For this review, take the finished solid that the model builds, in its own axes (mm). A direction names the side the tool comes from. Give positions to 0.01 mm unless a question says otherwise; leave off trailing zeros. Write each loop counter-clockwise with the first axis right and the second up, starting at its lowest first coordinate (ties: lowest second). Pieces come first, ordered by that corner, then holes. Notation, with made-up numbers: (85, 69) -> (143, 69) arc R26 cw to (143, 108) -> close; hole circle Ø7 at (18, -33). An arc over 180 degrees is marked (long way). Return JSON: item names as keys, results as strings.
from build123d import *

# Parameters (mm, degrees)
F2_R            = 12.5
F3_DEPTH        = 6
F5_DEPTH        = 68
F6_R            = 12.5
F7_DEPTH        = 12
F8_DEPTH        = 6
F12_D           = 8
F12_DEPTH       = 25
F12_CSINK_D     = 12
F12_CSINK_ANGLE = 60
F12_TIP         = 2.4034424761
F14_DEPTH       = 33
F15_R           = 9
F15_R_2         = 8.5
F16_DEPTH       = 6


with BuildPart() as f1:
    # F0 (on Front) → F1 (revolve)
    with BuildSketch(Plane.XZ):
        Polygon((0, 10), (0, 0), (86.0796358759, 0), (86.0796358759, 8), (85.0796358759, 9), (52.7846625228, 9), (52.7846625228, 8.5), (46, 8.5), (46, 10), align=None)
    revolve(axis=Axis((43.0398179379, 0, 0), (-1, 0, 0)))

    # F2 (on face) → F3 (join)
    with BuildSketch(Plane(origin=(0, 0, 0), x_dir=(0, -1, 0), z_dir=(-1, 0, 0))):
        Circle(F2_R)
    extrude(amount=F3_DEPTH)

    # F4 (on face) → F5 (join)
    with BuildSketch(Plane(origin=(-6, 0, 0), x_dir=(0, -1, 0), z_dir=(-1, 0, 0))):
        with BuildLine():
            Line((8.0269876576, 7.5211348309), (6.2374895659, 6.4879676259))
            ThreePointArc((6.2374895659, 6.4879676259), (4.5, 7.7942286341), (2.5, 8.6458082329))
            Line((2.5, 8.6458082329), (2.5, 10.7121426428))
            ThreePointArc((2.5, 10.7121426428), (0, 11), (-2.5, 10.7121426428))
            Line((-2.5, 10.7121426428), (-2.5, 8.6458082329))
            ThreePointArc((-2.5, 8.6458082329), (-4.5, 7.7942286341), (-6.2374895659, 6.4879676259))
            Line((-6.2374895659, 6.4879676259), (-8.0269876576, 7.5211348309))
            ThreePointArc((-8.0269876576, 7.5211348309), (-9.5262794416, 5.5), (-10.5269876576, 3.1910078119))
            Line((-10.5269876576, 3.1910078119), (-8.7374895659, 2.157840607))
            ThreePointArc((-8.7374895659, 2.157840607), (-9, 0), (-8.7374895659, -2.157840607))
            Line((-8.7374895659, -2.157840607), (-10.5269876576, -3.1910078119))
            ThreePointArc((-10.5269876576, -3.1910078119), (-9.5262794416, -5.5), (-8.0269876576, -7.5211348309))
            Line((-8.0269876576, -7.5211348309), (-6.2374895659, -6.4879676259))
            ThreePointArc((-6.2374895659, -6.4879676259), (-4.5, -7.7942286341), (-2.5, -8.6458082329))
            Line((-2.5, -8.6458082329), (-2.5, -10.7121426428))
            ThreePointArc((-2.5, -10.7121426428), (0, -11), (2.5, -10.7121426428))
            Line((2.5, -10.7121426428), (2.5, -8.6458082329))
            ThreePointArc((2.5, -8.6458082329), (4.5, -7.7942286341), (6.2374895659, -6.4879676259))
            Line((6.2374895659, -6.4879676259), (8.0269876576, -7.5211348309))
            ThreePointArc((8.0269876576, -7.5211348309), (9.5262794416, -5.5), (10.5269876576, -3.1910078119))
            Line((10.5269876576, -3.1910078119), (8.7374895659, -2.157840607))
            ThreePointArc((8.7374895659, -2.157840607), (9, 0), (8.7374895659, 2.157840607))
            Line((8.7374895659, 2.157840607), (10.5269876576, 3.1910078119))
            ThreePointArc((10.5269876576, 3.1910078119), (10.0928807369, 4.3742151788), (9.5262794416, 5.5))
            ThreePointArc((9.5262794416, 5.5), (8.8346218349, 6.5535835262), (8.0269876576, 7.5211348309))
        make_face()
    extrude(amount=F5_DEPTH)

    # F6 (on face) → F7 (cut)
    with BuildSketch(Plane(origin=(-6, 0, 0), x_dir=(0, -1, 0), z_dir=(-1, 0, 0))):
        Circle(F6_R)
        with BuildLine():
            ThreePointArc((2.5, 8.6458082329), (4.5, 7.7942286341), (6.2374895659, 6.4879676259))
            Line((6.2374895659, 6.4879676259), (8.0269876576, 7.5211348309))
            ThreePointArc((8.0269876576, 7.5211348309), (9.5262794416, 5.5), (10.5269876576, 3.1910078119))
            Line((10.5269876576, 3.1910078119), (8.7374895659, 2.157840607))
            ThreePointArc((8.7374895659, 2.157840607), (9, 0), (8.7374895659, -2.157840607))
            Line((8.7374895659, -2.157840607), (10.5269876576, -3.1910078119))
            ThreePointArc((10.5269876576, -3.1910078119), (9.5262794416, -5.5), (8.0269876576, -7.5211348309))
            Line((8.0269876576, -7.5211348309), (6.2374895659, -6.4879676259))
            ThreePointArc((6.2374895659, -6.4879676259), (4.5, -7.7942286341), (2.5, -8.6458082329))
            Line((2.5, -8.6458082329), (2.5, -10.7121426428))
            ThreePointArc((2.5, -10.7121426428), (0, -11), (-2.5, -10.7121426428))
            Line((-2.5, -10.7121426428), (-2.5, -8.6458082329))
            ThreePointArc((-2.5, -8.6458082329), (-4.5, -7.7942286341), (-6.2374895659, -6.4879676259))
            Line((-6.2374895659, -6.4879676259), (-8.0269876576, -7.5211348309))
            ThreePointArc((-8.0269876576, -7.5211348309), (-9.5262794416, -5.5), (-10.5269876576, -3.1910078119))
            Line((-10.5269876576, -3.1910078119), (-8.7374895659, -2.157840607))
            ThreePointArc((-8.7374895659, -2.157840607), (-9, 0), (-8.7374895659, 2.157840607))
            Line((-8.7374895659, 2.157840607), (-10.5269876576, 3.1910078119))
            ThreePointArc((-10.5269876576, 3.1910078119), (-9.5262794416, 5.5), (-8.0269876576, 7.5211348309))
            Line((-8.0269876576, 7.5211348309), (-6.2374895659, 6.4879676259))
            ThreePointArc((-6.2374895659, 6.4879676259), (-4.5, 7.7942286341), (-2.5, 8.6458082329))
            Line((-2.5, 8.6458082329), (-2.5, 10.7121426428))
            ThreePointArc((-2.5, 10.7121426428), (0, 11), (2.5, 10.7121426428))
            Line((2.5, 10.7121426428), (2.5, 8.6458082329))
        make_face(mode=Mode.SUBTRACT)
    extrude(amount=-F7_DEPTH, mode=Mode.SUBTRACT)

    # F6 (on face) → F8 (join)
    with BuildSketch(Plane(origin=(-6, 0, 0), x_dir=(0, -1, 0), z_dir=(-1, 0, 0))):
        Circle(F6_R)
        with BuildLine():
            ThreePointArc((2.5, 8.6458082329), (4.5, 7.7942286341), (6.2374895659, 6.4879676259))
            Line((6.2374895659, 6.4879676259), (8.0269876576, 7.5211348309))
            ThreePointArc((8.0269876576, 7.5211348309), (9.5262794416, 5.5), (10.5269876576, 3.1910078119))
            Line((10.5269876576, 3.1910078119), (8.7374895659, 2.157840607))
            ThreePointArc((8.7374895659, 2.157840607), (9, 0), (8.7374895659, -2.157840607))
            Line((8.7374895659, -2.157840607), (10.5269876576, -3.1910078119))
            ThreePointArc((10.5269876576, -3.1910078119), (9.5262794416, -5.5), (8.0269876576, -7.5211348309))
            Line((8.0269876576, -7.5211348309), (6.2374895659, -6.4879676259))
            ThreePointArc((6.2374895659, -6.4879676259), (4.5, -7.7942286341), (2.5, -8.6458082329))
            Line((2.5, -8.6458082329), (2.5, -10.7121426428))
            ThreePointArc((2.5, -10.7121426428), (0, -11), (-2.5, -10.7121426428))
            Line((-2.5, -10.7121426428), (-2.5, -8.6458082329))
            ThreePointArc((-2.5, -8.6458082329), (-4.5, -7.7942286341), (-6.2374895659, -6.4879676259))
            Line((-6.2374895659, -6.4879676259), (-8.0269876576, -7.5211348309))
            ThreePointArc((-8.0269876576, -7.5211348309), (-9.5262794416, -5.5), (-10.5269876576, -3.1910078119))
            Line((-10.5269876576, -3.1910078119), (-8.7374895659, -2.157840607))
            ThreePointArc((-8.7374895659, -2.157840607), (-9, 0), (-8.7374895659, 2.157840607))
            Line((-8.7374895659, 2.157840607), (-10.5269876576, 3.1910078119))
            ThreePointArc((-10.5269876576, 3.1910078119), (-9.5262794416, 5.5), (-8.0269876576, 7.5211348309))
            Line((-8.0269876576, 7.5211348309), (-6.2374895659, 6.4879676259))
            ThreePointArc((-6.2374895659, 6.4879676259), (-4.5, 7.7942286341), (-2.5, 8.6458082329))
            Line((-2.5, 8.6458082329), (-2.5, 10.7121426428))
            ThreePointArc((-2.5, 10.7121426428), (0, 11), (2.5, 10.7121426428))
            Line((2.5, 10.7121426428), (2.5, 8.6458082329))
        make_face(mode=Mode.SUBTRACT)
    extrude(amount=-F8_DEPTH)

    # F9 (on Front) → F10 (revolve)
    with BuildSketch(Plane.XZ):
        Polygon((-92, 0), (-74, 0), (-74, 2.157840607), (-74, 3.1910078119), (-74, 7.5211348309), (-74, 8.3), (-76, 8.3), (-76, 8.5), (-91, 8.5), (-92, 7.5), align=None)
    revolve(axis=Axis((-83, 0, 0), (1, 0, 0)))

    # F12
    with Locations(Plane.YZ.offset(86.0796358759)):
        with Locations((0, 0)):
            CounterSinkHole(F12_D / 2, F12_CSINK_D / 2, depth=F12_DEPTH, counter_sink_angle=F12_CSINK_ANGLE)
            with Locations((0, 0, -(F12_DEPTH + F12_TIP / 2))):  # 118° drill point
                Cone(0, F12_D / 2, F12_TIP, mode=Mode.SUBTRACT)

    # F13 (on face) → F14 (cut)
    with BuildSketch(Plane.YZ.offset(86.0796358759)):
        with BuildLine():
            Line((-2.5, 7), (0, 7))
            Line((0, 7), (2.5, 7))
            Line((2.5, 7), (2.5, 8.6458082329))
            ThreePointArc((2.5, 8.6458082329), (0, 9), (-2.5, 8.6458082329))
            Line((-2.5, 8.6458082329), (-2.5, 7))
        make_face()
    extrude(amount=-F14_DEPTH, mode=Mode.SUBTRACT)

    # F15 (on face) → F16 (join)
    with BuildSketch(Plane(origin=(52.7846625228, 0, 0), x_dir=(0, -1, 0), z_dir=(-1, 0, 0))):
        Circle(F15_R)
        Circle(F15_R_2, mode=Mode.SUBTRACT)
    extrude(amount=F16_DEPTH)


solid = f1.part
1. Add section A-A, the plane x = 73. State the section outline as (y, z) points, plus the area to 3 significant figures.
Results found:
{"outline": "(-2.5, 7) -> (-2.5, 8.65) arc R9 ccw (long way) to (2.5, 8.65) -> (2.5, 7) -> close; hole circle Ø8 at (0, 0)", "area": "195 mm²"}
2. To check wall thickness, follow probe 1 along Y at (x, z) = (75.75, 0); probe 2 along Z at (x, y) = (75.5, 0); probe 3 along Y at (x, z) = (-46, -6.75). State the ranges of each line that lie inside material, in increasing order.
Results found:
{"probe 1": "y = -9 to -4, 4 to 9", "probe 2": "z = -9 to -4, 4 to 7", "probe 3": "y = -8.69 to -6.69, -5.95 to 5.95, 6.69 to 8.69"}
3. For pin 1 (1.6 mm diameter, centred on y = 1, z = 8, fed in from +X); pin 2 (0.6 mm diameter, centred on y = 9.5, z = 0, fed in from -X); pin 3 (3 mm diameter, centred on x = 34.5, z = -4, fed in from +Y); pin 4 (6 mm diameter, centred on y = 9.5, z = 3, fed in from +X), all flat-tipped, find the tip position at first contact; note any pin that passes through.
Results found:
{"pin 1": "stops at x = 53.08", "pin 2": "stops at x = -6", "pin 3": "stops at y = 9.68", "pin 4": "stops at x = 86.08"}
4. Add section B-B, the plane x = -38.5. State the section outline as (y, z) points.
Results found:
{"outline": "(-10.53, -3.19) arc R11 ccw to (-8.03, -7.52) -> (-6.24, -6.49) arc R9 ccw to (-2.5, -8.65) -> (-2.5, -10.71) arc R11 ccw to (2.5, -10.71) -> (2.5, -8.65) arc R9 ccw to (6.24, -6.49) -> (8.03, -7.52) arc R11 ccw to (10.53, -3.19) -> (8.74, -2.16) arc R9 ccw to (8.74, 2.16) -> (10.53, 3.19) arc R11 ccw to (8.03, 7.52) -> (6.24, 6.49) arc R9 ccw to (2.5, 8.65) -> (2.5, 10.71) arc R11 ccw to (-2.5, 10.71) -> (-2.5, 8.65) arc R9 ccw to (-6.24, 6.49) -> (-8.03, 7.52) arc R11 ccw to (-10.53, 3.19) -> (-8.74, 2.16) arc R9 ccw to (-8.74, -2.16) -> close"}
5. For faces 4 (the cylindrical face through (71.697, 0.867, -3.905)), 5 (the cylindrical face through (-40.48, 9.51, -5.53)), 6 (the flat face through (-6, -5.5, -7.35)), list the 3-axis set-ups (+Z, -Z, +X, -X, +Y, -Y) from which the entire face can be reached by the end or side of a thin tool; tool diameter is ignored.
Results found:
{"face 4": "+X", "face 5": "-Z, -X, +Y", "face 6": "-X"}
6. Add section C-C, the plane x = 14.5. State the section outline as (y, z) points, plus the area to 3 significant figures.
Results found:
{"outline": "circle Ø20 at (0, 0)", "area": "314 mm²"}
7. The part is to be moulded in two halves that separate along Y. For faces 1 (the cylindrical face through (3, -9, 0)), 2 (the cylindrical face through (-3.042, -11.923, 3.755)), 3 (the cylindrical face through (2.958, -4.526, -7.779)), say which applies: +Y half, -Y half, draft (parallel to the pull), parting line (faces both ways), or undercut.
Results found:
{"face 1": "-Y half", "face 2": "parting line", "face 3": "undercut"}
